Autodesk Inventor part; units mm, degrees
ref_plane "YZ Plane" through (0, 0, 0) normal (1, 0, 0) x (0, 1, 0)
ref_plane "XZ Plane" through (0, 0, 0) normal (0, 1, 0) x (-1, 0, 0)
ref_plane "XY Plane" through (0, 0, 0) normal (0, 0, 1) x (1, 0, 0)
sketch "Sketch1" plane through (0, 0, 0) normal (0, 0, 1) x (1, 0, 0)
  line L0 (0, 0) -> (34, 0)
  line L1 (34, 0) -> (34, 153)
  line L2 (34, 153) -> (0, 153)
  line L3 (0, 153) -> (0, 0)
  circle A0 centre (17, 7) radius 1.5
  circle A1 centre (17, 146) radius 1.5
  point P0 (17, 153)
  point P1 (17, 0)
  dimension "d0" = 34
  dimension "d1" = 153
  dimension "d2" = 3
  dimension "d4" = 7
  dimension "d5" = 3
  dimension "d6" = 7
extrude "Extrusion1" add sketch "Sketch1" along normal blind 5
sketch "Sketch2" plane through (0, 0, 0) normal (0, 0, -1) x (-1, 0, 0)
  line L0 (0, 153) -> (0, 0)
  line L1 (0, 138) -> (-34, 138)
  line L2 (-34, 138) -> (-34, 15)
  line L3 (-34, 15) -> (0, 15)
  line L4 (0, 15) -> (0, 138)
  line L5 (-34, 0) -> (-34, 153)
  point P0 (0, 76.5)
  dimension "d10" = 123
extrude "Extrusion2" add sketch "Sketch2" along normal blind 5
sketch "Sketch7" plane through (0, 0, 5) normal (0, 0, 1) x (1, 0, 0)
  line L0 (29, 133) -> (0, 133)
  line L1 (0, 133) -> (0, 45)
  line L2 (0, 45) -> (29, 45)
  line L3 (29, 45) -> (29, 133)
  line L4 (34, 0) -> (34, 153)
  line L5 (34, 153) -> (0, 153)
  line L6 (0, 15) -> (34, 15)
  line L7 (34, 138) -> (0, 138)
  line L8 (0, 153) -> (0, 0)
  point P0 (29, 89)
  point P1 (17, 153)
  dimension "d33" = 30
  dimension "d34" = 5
  dimension "d35" = 5
extrude "Extrusion5" cut sketch "Sketch7" against normal through all contours L3 L2 L1 L0
properties part number "BP005" material "ABS Plastic"
Geometry: final body of the model. Coordinates: model frame, mm. A direction names the side the tool comes from. Give positions to 0.01 mm unless a question says otherwise; leave off trailing zeros. Write each loop counter-clockwise with the first axis right and the second up, starting at its lowest first coordinate (ties: lowest second). Pieces come first, ordered by that corner, then holes.
1. Section query A-A, the plane x = 17. Return loops of the section in (y, z).
2. Pin query (flat end, axial travel): P1, Ø2.5, axis at x = 23.5, z = -3, coming from the +Y side; P2, Ø7.5, axis at x = 12, y = 147, coming from the -Z side. Return the tip coordinate at first contact, or that it passes through.
3. Section query D-D, the plane x = 30.5. Return loops of the section in (y, z).
4. Draft query along X for faces 1 (the cylindrical face through (16.805, 144.513, 2.465)), 2 (the flat face through (0, 28, 0)), 3 (the flat face through (17, 0, 2)), 4 (the cylindrical face through (15.8, 7.9, 2.5)). Return one class per face: released by +X, released by -X, zero draft, split by the parting line, or undercut.
5. Reachability of faces 5 (the flat face through (0, 141, 2)), 6 (the flat face through (17, 9, 0)), 7 (the flat face through (17, 144, 0)), 8 (the flat face through (29, 88, 0)) from +Z, -Z, +X, -X, +Y, -Y: full face, straight path, thin tool, end or side. Return the list, or none.
6. Line query: probe 1 along Y at (x, z) = (17, 2.2); probe 2 along X at (y, z) = (146, 2.15); probe 3 along Y at (x, z) = (20, 3). Output: solid intervals per line, ascending.
7. Section query C-C, the plane z = 1.5. Return loops of the section in (x, y).
8. Section query B-B, the plane y = 7. Return loops of the section in (x, z).
Computed:
1. outline: (0, 0) - (5.5, 0) - (5.5, 5) - (0, 5) - close; (8.5, 0) - (15, 0) - (15, -5) - (45, -5) - (45, 5) - (8.5, 5) - close; (133, -5) - (138, -5) - (138, 0) - (144.5, 0) - (144.5, 5) - (133, 5) - close; (147.5, 0) - (153, 0) - (153, 5) - (147.5, 5) - close
2. P1: stops at y = 138
2. P2: stops at z = 0
3. outline: (0, 0) - (15, 0) - (15, -5) - (138, -5) - (138, 0) - (153, 0) - (153, 5) - (0, 5) - close
4. face 1: undercut
4. face 2: released by -X
4. face 3: zero draft
4. face 4: undercut
5. face 5: +Z, -Z, -X, +Y, -Y
5. face 6: -Z, +X, -X, -Y
5. face 7: -Z, +X, -X, +Y
5. face 8: +Z, -Z, -X
6. probe 1: y = 0 to 5.5, 8.5 to 45, 133 to 144.5, 147.5 to 153
6. probe 2: x = 0 to 15.5, 18.5 to 34
6. probe 3: y = 0 to 45, 133 to 153
7. outline: (0, 0) - (34, 0) - (34, 153) - (0, 153) - (0, 133) - (29, 133) - (29, 45) - (0, 45) - close; hole circle Ø3 at (17, 7); hole circle Ø3 at (17, 146)
8. outline: (0, 0) - (15.5, 0) - (15.5, 5) - (0, 5) - close; (18.5, 0) - (34, 0) - (34, 5) - (18.5, 5) - close
